```python
from build123d import *

# Parameters (mm, degrees)
ESQUISSE1_W             = 152.1
ESQUISSE1_H             = 25
ESQUISSE1_R             = 2.75
ESQUISSE1_R_2           = 2
BOSS_EXTRU_1_DEPTH      = 3
ESQUISSE3_R             = 6.1
ESQUISSE3_W             = 58.273048821
ESQUISSE3_H             = 11.159952414
ENL_V_MAT_EXTRU_2_DEPTH = 78.977892392


with BuildPart() as part:
    # Esquisse1 → Boss.-Extru.1 (new body)
    with BuildSketch(Plane(origin=(0, 0, 0), x_dir=(1, 0, 0), z_dir=(0, 1, 0))):
        with Locations((-0.495280426, -2.072980011)):
            Rectangle(ESQUISSE1_W, ESQUISSE1_H)
        with Locations(Location((65.554719574, -2.072980011, 0), (0, 0, 270))):
            Circle(ESQUISSE1_R, mode=Mode.SUBTRACT)
        with Locations(Location((-66.545280426, -2.072980011, 0), (0, 0, 270))):
            Circle(ESQUISSE1_R_2, mode=Mode.SUBTRACT)
    extrude(amount=BOSS_EXTRU_1_DEPTH)

    # Esquisse3 → Enlèv. mat.-Extru.2 (cut, through all)
    with BuildSketch(Plane(origin=(0, 0, 0), x_dir=(1, 0, 0), z_dir=(0, 1, 0))):
        with Locations(Location((-46.545280426, -2.072980011, 0), (0, 0, 270))):
            Circle(ESQUISSE3_R)
        with Locations(Location((-26.545280426, -2.072980011, 0), (0, 0, 270))):
            Circle(ESQUISSE3_R)
        with Locations((31.710873838, -7.652956218)):
            Rectangle(ESQUISSE3_W, ESQUISSE3_H)
    extrude(amount=ENL_V_MAT_EXTRU_2_DEPTH, mode=Mode.SUBTRACT)


solid = part.part
```
The listing builds one solid part. Answer for the finished solid, in the listing's coordinates (mm). A direction names the side the tool comes from. Coordinates: 2 decimals unless noted, no trailing zeros. Loops run counter-clockwise (first coordinate to the right, second up) from the corner with the lowest first, then second, coordinate; pieces in that order, holes last. Notation, with made-up numbers: M -0.5,40 L 16.5,40 A29 ccw 16.5,71 Z; hole C 16,-27.5 d11. An arc over 180 degrees is marked long. Answer as a JSON object with one key per item and string values. Group by question number.
Item 1: Consider L1, parallel to Z at x = 44, y = 2.75; L2, parallel to X at y = 1.9, z = 7.25; L3, parallel to X at y = 2.8, z = 8.25. Determine where each line is inside the solid, lowest interval first.
Item 2: Section A-A (x = 19.5) is taken. Write down the section's boundary in (y, z), and give its area (3 significant figures).
Item 3: Section B-B (z = 6.5) is taken. Write down the section's boundary in (x, y), and give its area (3 significant figures).
Item 4: Section C-C (y = 2.25) is taken. Write down the section's boundary in (x, z), and give its area (3 significant figures).
Item 5: Which of the six approach directions +Z, -Z, +X, -X, +Y, -Y give full straight-line access (tool end or side, diameter ignored) to faces 5 (the face through (31, 1, 2.073)), 6 (the face through (75.555, 1, 2))?
Item 6: Section D-D (x = -25) is taken. Write down the section's boundary in (y, z), and give its area (3 significant figures).
Item 7: Determine the mould class of faces 1 (the face through (2.574, 1, 8)), 2 (the face through (-76.545, 1, 2)), 3 (the face through (-2, 0, 2)), 4 (the face through (-20.497, 1.479, 1.279)) for opening direction X: +X half, -X half, draft (parallel to the pull), parting line (faces both ways), or undercut.
Solved:
{
 "1": {"L1": "z = -10.43 to 2.07, 13.23 to 14.57", "L2": "x = -76.55 to -49.77, -43.32 to -29.77, -23.32 to 2.57, 60.85 to 75.55", "L3": "x = -76.55 to 2.57, 60.85 to 75.55"},
 "2": {"outline": "M 0,-10.43 L 3,-10.43 L 3,2.07 L 0,2.07 Z; M 0,13.23 L 3,13.23 L 3,14.57 L 0,14.57 Z", "area": "41.5 mm2"},
 "3": {"outline": "M -76.55,0 L -50.74,0 L -50.74,3 L -76.55,3 Z; M -42.35,0 L -30.74,0 L -30.74,3 L -42.35,3 Z; M -22.35,0 L 2.57,0 L 2.57,3 L -22.35,3 Z; M 60.85,0 L 75.55,0 L 75.55,3 L 60.85,3 Z", "area": "231 mm2"},
 "4": {"outline": "M -76.55,-10.43 L 75.55,-10.43 L 75.55,14.57 L -76.55,14.57 Z; hole C -66.55,2.07 d4; hole C -46.55,2.07 d12.2; hole C -26.55,2.07 d12.2; hole M 2.57,2.07 L 60.85,2.07 L 60.85,13.23 L 2.57,13.23 Z; hole C 65.55,2.07 d5.5", "area": "2,880 mm2"},
 "5": {"face 5": "+Y, -Y", "face 6": "+Z, -Z, +X, +Y, -Y"},
 "6": {"outline": "M 0,-10.43 L 3,-10.43 L 3,-3.83 L 0,-3.83 Z; M 0,7.97 L 3,7.97 L 3,14.57 L 0,14.57 Z", "area": "39.6 mm2"},
 "7": {"face 1": "undercut", "face 2": "-X half", "face 3": "draft", "face 4": "undercut"}
}
